```python
from build123d import *

# Parameters (mm, degrees)
SKETCH2_R          = 3.6
CUT_EXTRUDE1_DEPTH = 10
SKETCH3_R          = 2.25
CUT_EXTRUDE2_DEPTH = 7.5
CHAMFER1_SIZE      = 1.5


with BuildPart() as part:
    # Sketch1 → Revolve1 (revolve)
    with BuildSketch(Plane(origin=(0, 0, 0), x_dir=(0, 0, -1), z_dir=(1, 0, 0)), mode=Mode.PRIVATE) as revolve1_sk:
        Polygon((0, 0), (-9.5, 0), (-9.5, 2), (-8, 2), (-8, 11), (-6.5, 11), (-6.5, 10.5), (0, 10.5), align=None)
    revolve(revolve1_sk.sketch.rotate(Axis((0, 0, 0), (0, 1, 0)), 180), axis=Axis((0, 0, 0), (0, 1, 0)))

    # Sketch2 → Cut-Extrude1 (cut)
    with BuildSketch(Plane.XZ):
        with Locations(Location((0, 0, 0), (0, 0, 270))):
            Circle(SKETCH2_R)
    extrude(amount=-CUT_EXTRUDE1_DEPTH, mode=Mode.SUBTRACT)

    # Sketch3 → Cut-Extrude2 (cut)
    with BuildSketch(Plane(origin=(0, 11, 0), x_dir=(1, 0, 0), z_dir=(0, 1, 0))):
        with Locations((-9.5, 0)):
            Circle(SKETCH3_R)
        with Locations((-5.923153118, 7.427399083)):
            Circle(SKETCH3_R)
        with Locations((2.113948873, 9.261815166)):
            Circle(SKETCH3_R)
        with Locations((8.559204245, 4.121895522)):
            Circle(SKETCH3_R)
        with Locations((8.559204245, -4.121895522)):
            Circle(SKETCH3_R)
        with Locations((2.113948873, -9.261815166)):
            Circle(SKETCH3_R)
        with Locations((-5.923153118, -7.427399083)):
            Circle(SKETCH3_R)
    extrude(amount=-CUT_EXTRUDE2_DEPTH, mode=Mode.SUBTRACT)

    # Chamfer1
    # the kernel refuses this chamfer: 1.5 mm, written as the material it takes off along each edge
    with BuildSketch(Plane(origin=(0, 3.5, 0), x_dir=(-0.43539008787732036, 0, 0.9002418960358263), z_dir=(-0.9002418960358263, 0, -0.43539008787732036))) as chamfer1_piece_1_section:
        Polygon((8, -CHAMFER1_SIZE), (8 - CHAMFER1_SIZE, 0), (8, 0), align=None)
    chamfer1_piece_1 = revolve(axis=Axis((0, 3.5, 0), (0, 1, 0)), revolution_arc=77.334522456, mode=Mode.PRIVATE)
    chamfer1_piece_1 = split(chamfer1_piece_1, bisect_by=Plane(origin=(1.717555098, 2, 7.525103296), z_dir=(0, 1, 0)), keep=Keep.TOP, mode=Mode.PRIVATE)
    chamfer1_piece_1 = chamfer1_piece_1 & Plane(origin=(2.113948873, 2.875825312, 9.261815166), x_dir=(1, 0, 0), z_dir=(0, 1, 0)) * Cylinder(2.25, 33, mode=Mode.PRIVATE)
    add(chamfer1_piece_1, mode=Mode.SUBTRACT)
    with BuildSketch(Plane(origin=(0, 3.5, 0), x_dir=(-0.975298735779407, 0, 0.2208899635272972), z_dir=(-0.2208899635272972, 0, -0.975298735779407))) as chamfer1_piece_2_section:
        Polygon((8, -CHAMFER1_SIZE), (8 - CHAMFER1_SIZE, 0), (8, 0), align=None)
    chamfer1_piece_2 = revolve(axis=Axis((0, 3.5, 0), (0, 1, 0)), revolution_arc=77.334522456, mode=Mode.PRIVATE)
    chamfer1_piece_2 = split(chamfer1_piece_2, bisect_by=Plane(origin=(-4.812484572, 2, 6.034663839), z_dir=(0, 1, 0)), keep=Keep.TOP, mode=Mode.PRIVATE)
    chamfer1_piece_2 = chamfer1_piece_2 & Plane(origin=(-5.923153118, 2.875825413, 7.427399083), x_dir=(1, 0, 0), z_dir=(0, 1, 0)) * Cylinder(2.25, 32, mode=Mode.PRIVATE)
    add(chamfer1_piece_2, mode=Mode.SUBTRACT)
    with BuildSketch(Plane(origin=(0, 3.5, 0), x_dir=(-0.7807875431710312, 0, -0.624796616851392), z_dir=(0.624796616851392, 0, -0.7807875431710312))) as chamfer1_piece_3_section:
        Polygon((8, -CHAMFER1_SIZE), (8 - CHAMFER1_SIZE, 0), (8, 0), align=None)
    chamfer1_piece_3 = revolve(axis=Axis((0, 3.5, 0), (0, 1, 0)), revolution_arc=77.334522456, mode=Mode.PRIVATE)
    chamfer1_piece_3 = split(chamfer1_piece_3, bisect_by=Plane(origin=(-7.718624937, 2, -1.33e-07), z_dir=(0, 1, 0)), keep=Keep.TOP, mode=Mode.PRIVATE)
    chamfer1_piece_3 = chamfer1_piece_3 & Plane(origin=(-9.5, 2.875824947, 0), x_dir=(1, 0, 0), z_dir=(0, 1, 0)) * Cylinder(2.25, 32, mode=Mode.PRIVATE)
    add(chamfer1_piece_3, mode=Mode.SUBTRACT)
    with BuildSketch(Plane(origin=(0, 3.5, 0), x_dir=(0.0016725946084597224, 0, -0.9999986012126596), z_dir=(0.9999986012126596, 0, 0.0016725946084597224))) as chamfer1_piece_4_section:
        Polygon((8, -CHAMFER1_SIZE), (8 - CHAMFER1_SIZE, 0), (8, 0), align=None)
    chamfer1_piece_4 = revolve(axis=Axis((0, 3.5, 0), (0, 1, 0)), revolution_arc=77.334522456, mode=Mode.PRIVATE)
    chamfer1_piece_4 = split(chamfer1_piece_4, bisect_by=Plane(origin=(-4.81248369, 2, -6.034664462), z_dir=(0, 1, 0)), keep=Keep.TOP, mode=Mode.PRIVATE)
    chamfer1_piece_4 = chamfer1_piece_4 & Plane(origin=(-5.923153118, 2.875825391, -7.427399083), x_dir=(1, 0, 0), z_dir=(0, 1, 0)) * Cylinder(2.25, 32, mode=Mode.PRIVATE)
    add(chamfer1_piece_4, mode=Mode.SUBTRACT)
    with BuildSketch(Plane(origin=(0, 3.5, 0), x_dir=(0.782873234533069, 0, -0.6221812426067909), z_dir=(0.6221812426067909, 0, 0.782873234533069))) as chamfer1_piece_5_section:
        Polygon((8, -CHAMFER1_SIZE), (8 - CHAMFER1_SIZE, 0), (8, 0), align=None)
    chamfer1_piece_5 = revolve(axis=Axis((0, 3.5, 0), (0, 1, 0)), revolution_arc=77.334522456, mode=Mode.PRIVATE)
    chamfer1_piece_5 = split(chamfer1_piece_5, bisect_by=Plane(origin=(1.717556284, 2, -7.525103041), z_dir=(0, 1, 0)), keep=Keep.TOP, mode=Mode.PRIVATE)
    chamfer1_piece_5 = chamfer1_piece_5 & Plane(origin=(2.113948873, 2.875825447, -9.261815166), x_dir=(1, 0, 0), z_dir=(0, 1, 0)) * Cylinder(2.25, 32, mode=Mode.PRIVATE)
    add(chamfer1_piece_5, mode=Mode.SUBTRACT)
    with BuildSketch(Plane(origin=(0, 3.5, 0), x_dir=(0.9745543611505972, 0, 0.22415128186640224), z_dir=(-0.22415128186640224, 0, 0.9745543611505972))) as chamfer1_piece_6_section:
        Polygon((8, -CHAMFER1_SIZE), (8 - CHAMFER1_SIZE, 0), (8, 0), align=None)
    chamfer1_piece_6 = revolve(axis=Axis((0, 3.5, 0), (0, 1, 0)), revolution_arc=77.334522456, mode=Mode.PRIVATE)
    chamfer1_piece_6 = split(chamfer1_piece_6, bisect_by=Plane(origin=(6.9542413, 2, -3.34898542), z_dir=(0, 1, 0)), keep=Keep.TOP, mode=Mode.PRIVATE)
    chamfer1_piece_6 = chamfer1_piece_6 & Plane(origin=(8.559204245, 2.875825426, -4.121895522), x_dir=(1, 0, 0), z_dir=(0, 1, 0)) * Cylinder(2.25, 32, mode=Mode.PRIVATE)
    add(chamfer1_piece_6, mode=Mode.SUBTRACT)
    with BuildSketch(Plane(origin=(0, 3.5, 0), x_dir=(0.43237617653563165, 0, 0.9016933192413196), z_dir=(-0.9016933192413196, 0, 0.43237617653563165))) as chamfer1_piece_7_section:
        Polygon((8, -CHAMFER1_SIZE), (8 - CHAMFER1_SIZE, 0), (8, 0), align=None)
    chamfer1_piece_7 = revolve(axis=Axis((0, 3.5, 0), (0, 1, 0)), revolution_arc=77.334522456, mode=Mode.PRIVATE)
    chamfer1_piece_7 = split(chamfer1_piece_7, bisect_by=Plane(origin=(6.954240779, 2, 3.348986578), z_dir=(0, 1, 0)), keep=Keep.TOP, mode=Mode.PRIVATE)
    chamfer1_piece_7 = chamfer1_piece_7 & Plane(origin=(8.559204245, 2.875825449, 4.121895522), x_dir=(1, 0, 0), z_dir=(0, 1, 0)) * Cylinder(2.25, 32, mode=Mode.PRIVATE)
    add(chamfer1_piece_7, mode=Mode.SUBTRACT)


solid = part.part
```
Source: CAD feature listing. Evaluate the final solid. Frame: model axes, mm. A direction names the side the tool comes from. Round coordinates to 2 decimals unless told otherwise and drop trailing zeros. Loops run counter-clockwise (first coordinate to the right, second up) from the corner with the lowest first, then second, coordinate; pieces in that order, holes last.
(1) Section query B-B (y = 8.5). Output: boundary loops of the cut face in (x, z).
From the geometry:
outline: (-7.85, -1.53) arc R8 ccw to (-6.09, -5.18) arc R2.25 cw to (-3.7, -7.09) arc R8 ccw to (0.25, -8) arc R2.25 cw to (3.24, -7.31) arc R8 ccw to (6.41, -4.79) arc R2.25 cw to (7.74, -2.03) arc R8 ccw to (7.74, 2.03) arc R2.25 cw to (6.41, 4.79) arc R8 ccw to (3.24, 7.31) arc R2.25 cw to (0.25, 8) arc R8 ccw to (-3.7, 7.09) arc R2.25 cw to (-6.09, 5.18) arc R8 ccw to (-7.85, 1.53) arc R2.25 cw to start; hole circle Ø7.2 at (0, 0)
(2) Material intervals for probe 1 along X at (y, z) = (4.25, 0); probe 2 along X at (y, z) = (10.85, 0); probe 3 along Y at (x, z) = (-1.75, -4.75), sorted ascending.
From the geometry:
probe 1: x = -7.25 to -3.6, 3.6 to 8
probe 2: x = -7.25 to -6.5, 6.5 to 8
probe 3: y = 0 to 10.5
(3) Access query for faces 4 (the flat face through (7, 2, 4.3)), 5 (the cylindrical face through (4.97, 6.56, 6.27)), 6 (the cylindrical face through (-7.195, 6.563, -3.497)), 7 (the conical face through (1.734, 2.297, -7.505)). Directions: +Z, -Z, +X, -X, +Y, -Y. A direction counts if a zero-diameter tool reaches every point of the face in a straight line with its end or side. Return the directions, or none.
From the geometry:
face 4: +Y
face 5: +Z, +X, +Y
face 6: -Z, -X, +Y
face 7: -Z, +Y
(4) Section query A-A (z = 0). Output: boundary loops of the cut face in (x, y), and give its area (3 significant figures).
From the geometry:
outline: (-9.5, 0) - (-3.6, 0) - (-3.6, 10) - (3.6, 10) - (3.6, 0) - (9.5, 0) - (9.5, 2) - (8, 2) - (8, 11) - (6.5, 11) - (6.5, 10.5) - (-6.5, 10.5) - (-6.5, 11) - (-7.25, 11) - (-7.25, 2.75) - (-8, 2) - (-9.5, 2) - close
area: 97.0 mm2
(5) Pull-direction query (Z, two-part tool) for faces 1 (the cylindrical face through (9.274, 1.014, 2.059)), 2 (the cylindrical face through (-7.25, 6.56, 0.02)), 3 (the cylindrical face through (5.01, 6.563, -6.237)); classes: +Z half, -Z half, draft (parallel to the pull), parting line (faces both ways), or undercut.
From the geometry:
face 1: parting line
face 2: undercut
face 3: -Z half
(6) Section query C-C (x = 0). Output: boundary loops of the cut face in (y, z), and give its area (4 significant figures).
From the geometry:
outline: (0, -9.5) - (2, -9.5) - (2, -8) - (11, -8) - (11, -6.5) - (10.5, -6.5) - (10.5, 6.5) - (11, 6.5) - (11, 8) - (2, 8) - (2, 9.5) - (0, 9.5) - (0, 3.6) - (10, 3.6) - (10, -3.6) - (0, -3.6) - close
area: 103.5 mm2
(7) Contact query for flat-ended pins moving along their axis: pin 1 Ø5 at (x, z) = (-6.5, -2) entering from -Y; pin 2 Ø8 at (x, z) = (0, 0) entering from +Y; pin 3 Ø4 at (x, y) = (7, 9) entering from +Z (3 decimals); pin 4 Ø2 at (x, z) = (-1.5, 1) entering from -Y. Output: stop coordinate, or through.
From the geometry:
pin 1: stops at y = 0
pin 2: stops at y = 10.5
pin 3: stops at z = 6.245
pin 4: stops at y = 10
(8) Section query D-D (x = -2.5). Output: boundary loops of the cut face in (y, z).
From the geometry:
outline: (0, -9.17) - (2, -9.17) - (2, -7.6) - (11, -7.6) - (11, -6) - (10.5, -6) - (10.5, 6) - (11, 6) - (11, 7.6) - (2, 7.6) - (2, 9.17) - (0, 9.17) - (0, 2.59) - (10, 2.59) - (10, -2.59) - (0, -2.59) - close
